Design review of the part built by this model. Coordinates are the model's own, in mm. A direction names the side the tool comes from. Coordinates: 2 decimals unless noted, no trailing zeros. Write each loop counter-clockwise with the first axis right and the second up, starting at its lowest first coordinate (ties: lowest second). Pieces come first, ordered by that corner, then holes. Notation, with made-up numbers: (-28.75, -36) - (-14.75, -36) arc R13 cw to (-14.75, -27) - close; hole circle Ø10 at (65.5, -25.5). An arc over 180 degrees is marked (long way). Answer as CSV lines item,"result". Start each with the question number.
Q1. We need section C-C (y = 42). Write out the cut boundary in (x, z), plus the area to 3 significant figures.
Q2. Clearance check with flat-ended pins moving along their axes: pin 1 (3 mm diameter, centred on y = -2, z = 2.5, fed in from +X); pin 2 (2 mm diameter, centred on x = -4, z = -2.5, fed in from +Y); pin 3 (1.5 mm diameter, centred on x = -4.5, y = 45, fed in from +Z). State where each tip first meets the part, or that it passes through.
Q3. We need section D-D (z = 4.5). Write out the cut boundary in (x, y), plus the area to 3 significant figures.
Q4. For line 1 along Y through (x, z) = (1, 5.5); line 2 along Y through (x, z) = (-5, -3.75); line 3 along Y through (x, z) = (-2, -1), list the stretches that pass through material, from the lowest coordinate up. Write a range as [from, to].
Q5. Machinability: for faces 1 (the face through (-6.2, -4.95, -1.38)), 2 (the face through (-2, 50.902, -3)), which of the approach directions +Z, -Z, +X, -X, +Y, -Y give a long, thin tool a straight path to every point of the face, cutting with its end or side? Answer none if there is none.
Q6. Mouldability with a two-part tool opening along Y and no side actions: class faces 3 (the face through (0, -62.395, 0)), 4 (the face through (0, 62.395, 0)), 5 (the face through (-0.526, -58.183, 0.089)), 6 (the face through (-1.93, 56.73, -2.52)) as pulls with the +Y half, pulls with the -Y half, needs draft (parallel to the pull), parting line crosses it, or undercut.
Q7. We need section A-A (x = 0). State how many separate pieces and enclosed holes the cut face has, plus the area to 3 significant figures.
from build123d import *

# Parameters (mm, degrees)
SKETCH1_R           = 6.35
BOSS_EXTRUDE1_DEPTH = 62.3951
SKETCH3_OUTSIDE_W   = 39.916
SKETCH3_OUTSIDE_H   = 39.916
SKETCH3_OUTSIDE_R   = 3.175
CUT_EXTRUDE1_DEPTH  = 11.4935
SKETCH7_R           = 1.7526
CUT_EXTRUDE3_DEPTH  = 9.525
SKETCH10_R          = 2.3495
CUT_EXTRUDE6_DEPTH  = 6.35


with BuildPart() as part:
    # Sketch1 → Boss-Extrude1 (new, symmetric)
    with BuildSketch(Plane(origin=(0, 0, 0), x_dir=(1, 0, 0), z_dir=(0, 1, 0))):
        with Locations(Location((0, 0, 0), (0, 0, 270))):
            Circle(SKETCH1_R)
    extrude(amount=BOSS_EXTRUDE1_DEPTH, both=True)

    # Sketch3 outside → Cut-Extrude1 (cut)
    with BuildSketch(Plane(origin=(0, 62.3951, 0), x_dir=(1, 0, 0), z_dir=(0, 1, 0))):
        Rectangle(SKETCH3_OUTSIDE_W, SKETCH3_OUTSIDE_H)
        with Locations(Location((0, 0, 0), (0, 0, 270))):
            Circle(SKETCH3_OUTSIDE_R, mode=Mode.SUBTRACT)
    extrude(amount=-CUT_EXTRUDE1_DEPTH, mode=Mode.SUBTRACT)

    # Sketch7 → Cut-Extrude3 (cut, symmetric)
    with BuildSketch(Plane.XY):
        with Locations(Location((0, -59.8551, 0), (0, 0, 89.99999997))):
            Circle(SKETCH7_R)
    extrude(amount=CUT_EXTRUDE3_DEPTH, both=True, mode=Mode.SUBTRACT)

    # Sketch10 → Cut-Extrude6 (cut, symmetric)
    with BuildSketch(Plane.XY):
        with Locations(Location((0, -6.2484, 0), (0, 0, 90.000000013))):
            Circle(SKETCH10_R)
    extrude(amount=CUT_EXTRUDE6_DEPTH, both=True, mode=Mode.SUBTRACT)


solid = part.part
Results list:
1,outline,"circle Ø12.7 at (0, 0)"
1,area,"127 mm2"
2,pin 1,"stops at x = 6.27"
2,pin 2,"stops at y = 50.9"
2,pin 3,"stops at z = 5.12"
3,outline,"(-4.48, -62.4) - (4.48, -62.4) - (4.48, 50.9) - (-4.48, 50.9) - close; hole circle Ø4.7 at (0, -6.25); hole circle Ø3.51 at (0, -59.86)"
3,area,"988 mm2"
4,line 1,"y = [-62.4, -61.29], [-58.42, -8.37], [-4.12, 50.9]"
4,line 2,"y = [-62.4, 50.9]"
4,line 3,"y = [-62.4, -7.48], [-5.02, 62.4]"
5,face 1,"+Y, -Y"
5,face 2,"+Y"
6,face 3,"pulls with the -Y half"
6,face 4,"pulls with the +Y half"
6,face 5,"undercut"
6,face 6,"needs draft"
7,separate pieces,"3"
7,enclosed holes,"0"
7,area,"1,410 mm2"
